```python
from build123d import *

# Parameters (mm, degrees)
F0_R     = 10.5
F1_DEPTH = 2
F0_R_2   = 12.5
F2_DEPTH = 4
F3_W     = 3
F3_H     = 7
F4_DEPTH = 7
F6_R     = 3
F5_R     = 1.5
F7_DEPTH = 25
F8_R     = 1.99999
F9_R     = 1


# Not quite as in the source:
# - a fillet or chamfer is up to 0.001 mm smaller than in the source, because OpenCascade refuses the exact size


with BuildPart() as f1:
    # F0 (on Top) → F1 (new body)
    with BuildSketch(Plane.XY):
        Circle(F0_R)
    extrude(amount=-F1_DEPTH)

    # F0 (on Top) → F2 (join)
    with BuildSketch(Plane.XY):
        Circle(F0_R_2)
        Circle(F0_R, mode=Mode.SUBTRACT)
        Circle(F0_R)
    extrude(amount=F2_DEPTH)

    # F3 (on face) → F4 (join)
    with BuildSketch(Plane.XY.offset(4)):
        Rectangle(F3_W, F3_H)
    extrude(amount=F4_DEPTH)

    # F6
    f6_edges = [f1.edges().sort_by_distance(p)[0] for p in [
        (0, -3.5, 11),
        (0, 3.5, 11),
    ]]
    fillet(f6_edges, radius=F6_R)

    # F5 (on face) → F7 (cut)
    with BuildSketch(Plane.YZ.offset(1.5)):
        with Locations((0, 7.438564696)):
            Circle(F5_R)
    extrude(amount=-F7_DEPTH, mode=Mode.SUBTRACT)

    # F8 (radius 2 in the source; OpenCascade refuses exactly that, so slightly less here)
    f8_edges = [f1.edges().sort_by_distance(p)[0] for p in [
        (-10.5, 0, -2),
    ]]
    fillet(f8_edges, radius=F8_R)

    # F9
    f9_edges = [f1.edges().sort_by_distance(p)[0] for p in [
        (12.5, 0, 2),
        (-12.5, 0, 0),
        (-12.5, 0, 4),
    ]]
    fillet(f9_edges, radius=F9_R)


solid = f1.part
```
Could you check a few things on this model? Use its own coordinates, in mm. A direction names the side the tool comes from. Give positions to 0.01 mm unless a question says otherwise; leave off trailing zeros. Loops run counter-clockwise (first coordinate to the right, second up) from the corner with the lowest first, then second, coordinate; pieces in that order, holes last. Notation, with made-up numbers: (-17, 6) - (22, 6) arc R31 ccw to (22, 44) - close; hole circle Ø5 at (-27, 22.5). An arc over 180 degrees is marked (long way). Use one line per item in the form item = value.
1. Thinking about a two-plate mould opening in Y: for faces 6 (the face through (0.021, -0.195, 8.926)), 7 (the face through (1.5, 1, 6)), 8 (the face through (0, 3.5, 6)), which applies, released by +Y, released by -Y, zero draft, split by the parting line, or undercut?
Response values:
face_6 = undercut
face_7 = zero draft
face_8 = released by +Y
2. I'm going to push flat-ended pins straight in: pin 1 Ø2 at (y, z) = (1.5, 8.5) entering from +X; pin 2 Ø8 at (x, y) = (3.5, -4.5) entering from +Z; pin 3 Ø1.5 at (x, y) = (7, -9.5) entering from +Z; pin 4 Ø5 at (y, z) = (0.5, 0) entering from +X. Where does each tip first touch, or does it pass through?
Response values:
pin_1 = 1.5
pin_2 = 10.95
pin_3 = 4
pin_4 = 12.5
3. On a 3-axis mill with a long thin cutter (end or side, diameter ignored), from which of +Z, -Z, +X, -X, +Y, -Y can I reach the whole of each face in a straight line? I mean faces 1 (the face through (-1.5, 1, 6)), 2 (the face through (0, -3.5, 6)), 3 (the face through (10.2, -3.4, 0)), 4 (the face through (0, 0, -2)), 5 (the face through (0, 0, 11)). Say none if no direction works.
Response values:
face_1 = +Z, -X, +Y, -Y
face_2 = +Z, +X, -X, -Y
face_3 = -Z
face_4 = -Z, +X, -X, +Y, -Y
face_5 = +Z, +X, -X, +Y, -Y
4. I need wall thicknesses on probe 1 along Z at (x, y) = (0.1, 0); probe 2 along X at (y, z) = (0, 10); probe 3 along Z at (x, y) = (5, -0.5). Which ranges of each line are inside material? Lowest first, please.
Response values:
probe_1 = -2 to 5.94, 8.94 to 11
probe_2 = -1.5 to 1.5
probe_3 = -2 to 4
5. I want a section at B-B (z = 4.75). Please give me the cut outline in (x, y), and give its area (3 significant figures).
Response values:
outline = (-1.5, -3.5) - (1.5, -3.5) - (1.5, 3.5) - (-1.5, 3.5) - close
area = 21.0 mm²
